Work out the finished part from the listing and answer in its coordinate system (mm). Coordinates: 2 decimals unless noted, no trailing zeros. Loops run counter-clockwise (first coordinate to the right, second up) from the corner with the lowest first, then second, coordinate; pieces in that order, holes last. Notation, with made-up numbers: (-16, 58) -> (43, 58) arc R21 ccw to (43, 83) -> close; hole circle Ø10 at (38.5, 45). An arc over 180 degrees is marked (long way). Use a Markdown table: item, result.
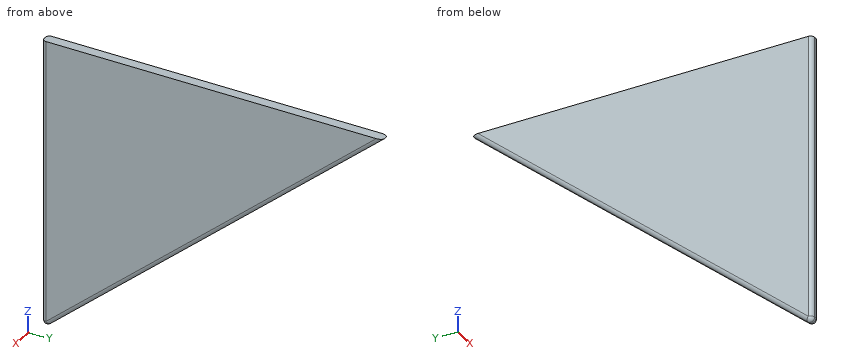
Autodesk Inventor part; units mm, degrees
ref_plane "Work Plane1" through (31.75, 0, 0) normal (1, 0, 0) x (0, 1, 0)
ref_plane "XZ Plane" through (0, 0, 0) normal (0, 1, 0) x (-1, 0, 0)
ref_plane "XY Plane" through (0, 0, 0) normal (0, 0, 1) x (1, 0, 0)
sketch "Sketch1" plane through (0, 0, 0) normal (1, 0, 0) x (0, 1, 0)
  line L0 (0, 0) -> (0, -1828.8)
  line L1 (0, -1828.8) -> (2133.6, 0)
  line L2 (2133.6, 0) -> (0, 0)
  dimension "d2" = 1828.8
  dimension "d3" = 2133.6
extrude "Extrusion1" add sketch "Sketch1" along normal blind 63.5
ref_plane "Work Plane1" through (31.75, 0, 0) normal (1, 0, 0) x (0, 1, 0)
fillet "Fillet4" radius 25.4 1 edges at (63.5, 1066.8, -914.4)
fillet "Fillet5" radius 25.4 1 edges at (0, 1066.8, -914.4)
fillet "Fillet6" radius 25.4 5 edges at (56.0605, 0, -1819.0016) (31.75, 0, -1828.8) (7.4395, 0, -1819.0016) (0, 0, -897.6731) (63.5, 0, -897.6731)
properties part number "RedSail-ver1-1111-2021"
Q1. Section A-A on x = 15.5 is taken. Determine the outline of the cut face in (y, z), and give its area (3 significant figures).
Solved:
| item | result |
|---|---|
| outline | (2.01, -1773.57) arc R23.39 ccw to (40.62, -1791.33) -> (2130.51, 0) -> (2.01, 0) -> close |
| area | 1,940,000 mm² |
Q2. Consider line 1 (Y direction, x = 38.5, z = -1277.5); line 2 (Z direction, x = 57.5, y = 1802); line 3 (Y direction, x = 8, z = -1456). Determine where each line is inside the solid, lowest interval first. Write a range as [from, to].
Solved:
| item | result |
|---|---|
| line 1 | [0, 643.18] |
| line 2 | [-272.37, 0] |
| line 3 | [6.9, 424.34] |
Q3. Given pin 1 Ø8 at (x, z) = (55.5, -1587.5) entering from -Y; pin 2 Ø1 at (x, z) = (18, -566) entering from +Y; pin 3 Ø1.5 at (x, y) = (45.5, 1605.5) entering from +Z; pin 4 Ø12 at (x, y) = (46, 418) entering from -Z, each flat-ended and moving along its own axis, determine where each tip first touches the part or whether it passes through.
Solved:
| item | result |
|---|---|
| pin 1 | y = 3.82 |
| pin 2 | y = 1472.2 |
| pin 3 | z = 0 |
| pin 4 | z = -1474.45 |
